Source: CAD feature listing. Evaluate the final solid. Frame: model axes, mm. A direction names the side the tool comes from. Round coordinates to 2 decimals unless told otherwise and drop trailing zeros. Answer in a Markdown table with one row per item. Add a question column.
```python
from build123d import *

# Parameters (mm, degrees)
ESQUISSE2_R                  = 39.5
BOSS_EXTRU_1_DEPTH           = 1
ESQUISSE4_R                  = 41.25
BOSS_EXTRU_2_DEPTH           = 1
ESQUISSE5_R                  = 42
BOSS_EXTRU_3_DEPTH           = 7
ESQUISSE6_R                  = 35
BOSS_EXTRU_4_DEPTH           = 7
BOSS_EXTRU_7_DEPTH           = 3
R_P_TITION_START             = -52
R_P_TITION_CIRCULAIRE1_DEPTH = 3
ESQUISSE8_R                  = 15
BOSS_EXTRU_8_DEPTH           = 10
ESQUISSE9_W                  = 24
ESQUISSE9_H                  = 40
BOSS_EXTRU_9_DEPTH           = 42
BOSS_EXTRU_10_DEPTH          = 24
ESQUISSE11_R                 = 15
BOSS_EXTRU_11_DEPTH          = 10
BOSS_EXTRU_12_START          = 10
ESQUISSE12_R                 = 15
BOSS_EXTRU_12_DEPTH          = 10


# Read off the part's stored shape, not the designer's step: Répétition circulaire1
with BuildPart() as part:
    # Esquisse1 → Révolution1 (revolve)
    with BuildSketch(Plane.XY):
        with BuildLine():
            Line((0, 0), (-35, 0))
            ThreePointArc((-35, 0), (-39.657515479, -9.46062113), (-40, -20))
            Line((-40, -20), (0, -20))
            Line((0, -20), (0, 0))
        make_face()
    revolve(axis=Axis((0, 0, 0), (0, -1, 0)))

    # Esquisse2 → Boss.-Extru.1 (add)
    with BuildSketch(Plane.XZ.offset(20)):
        Circle(ESQUISSE2_R)
    extrude(amount=BOSS_EXTRU_1_DEPTH)

    # Esquisse3 → Révolution2 (revolve)
    with BuildSketch(Plane(origin=(0, 0, 0), x_dir=(0, 0, -1), z_dir=(1, 0, 0)), mode=Mode.PRIVATE) as r_volution2_sk:
        with BuildLine():
            Line((0, -21), (-40, -21))
            ThreePointArc((-40, -21), (-42.384109041, -30.861589096), (-42, -41))
            Line((-42, -41), (0, -41))
            Line((0, -41), (0, -21))
        make_face()
    revolve(r_volution2_sk.sketch.rotate(Axis((0, -21, 0), (0, -1, 0)), 90), axis=Axis((0, -21, 0), (0, -1, 0)))

    # Esquisse4 → Boss.-Extru.2 (add)
    with BuildSketch(Plane.XZ.offset(41)):
        with Locations(Location((0, 0, 0), (0, 0, 270))):
            Circle(ESQUISSE4_R)
    extrude(amount=BOSS_EXTRU_2_DEPTH)

    # Esquisse5 → Boss.-Extru.3 (add)
    with BuildSketch(Plane.XZ.offset(42)):
        with Locations(Location((0, 0, 0), (0, 0, 270))):
            Circle(ESQUISSE5_R)
    extrude(amount=BOSS_EXTRU_3_DEPTH)

    # Esquisse6 → Boss.-Extru.4 (add)
    with BuildSketch(Plane.XZ.offset(49)):
        with Locations(Location((0, 0, 0), (0, 0, 270))):
            Circle(ESQUISSE6_R)
    extrude(amount=BOSS_EXTRU_4_DEPTH)

    # Esquisse7 → Boss.-Extru.7 (add)
    with BuildSketch(Plane.XZ.offset(49)):
        Polygon((39.629367086, -1.94603582), (40.75, 0.005042677), (39.620632914, 1.951078497), (37.370632914, 1.94603582), (36.25, -0.005042677), (37.379367086, -1.951078497), align=None)
        Polygon((39.045525279, 0.94978706), (37.950222917, 0.94733228), (37.404697638, -0.00245478), (37.954474721, -0.94978706), (39.049777083, -0.94733228), (39.595302362, 0.00245478), align=None, mode=Mode.SUBTRACT)
    extrude(amount=BOSS_EXTRU_7_DEPTH)

    # Répétition circulaire1 outline → Répétition circulaire1 (add)
    # profile 1 of 7: a face of its own
    with BuildSketch(Plane(origin=(0, 0, 0), x_dir=(1, 0, 0), z_dir=(0, 1, 0)).offset(R_P_TITION_START)):
        Polygon((29.398249326, -26.646139076), (27.810824779, -25.051583107), (25.636186529, -25.629055107), (25.048972826, -27.801083076), (26.636397373, -29.395639044), (28.811035623, -28.818167044), align=None)
        Polygon((28.282227258, -26.9424971), (27.996371011, -27.999842595), (26.937754829, -28.28095657), (26.164994893, -27.504725051), (26.45085114, -26.447379557), (27.509467323, -26.166265581), align=None, mode=Mode.SUBTRACT)
    # profile 2 of 7: a face of its own
    with BuildSketch(Plane(origin=(0, 0, 0), x_dir=(1, 0, 0), z_dir=(0, 1, 0)).offset(R_P_TITION_START)):
        Polygon((26.646139076, 29.398249326), (25.051583107, 27.810824779), (25.629055107, 25.636186529), (27.801083076, 25.048972826), (29.395639044, 26.636397373), (28.818167044, 28.811035623), align=None)
        Polygon((26.9424971, 28.282227258), (27.999842595, 27.996371011), (28.28095657, 26.937754829), (27.504725051, 26.164994893), (26.447379557, 26.45085114), (26.166265581, 27.509467323), align=None, mode=Mode.SUBTRACT)
    # profile 3 of 7: a face of its own
    with BuildSketch(Plane(origin=(0, 0, 0), x_dir=(1, 0, 0), z_dir=(0, 1, 0)).offset(R_P_TITION_START)):
        Polygon((-1.94603582, 39.629367086), (-1.951078497, 37.379367086), (-0.005042677, 36.25), (1.94603582, 37.370632914), (1.951078497, 39.620632914), (0.005042677, 40.75), align=None)
        Polygon((-0.94733228, 39.049777083), (0.00245478, 39.595302362), (0.94978706, 39.045525279), (0.94733228, 37.950222917), (-0.00245478, 37.404697638), (-0.94978706, 37.954474721), align=None, mode=Mode.SUBTRACT)
    # profile 4 of 7: a face of its own
    with BuildSketch(Plane(origin=(0, 0, 0), x_dir=(1, 0, 0), z_dir=(0, 1, 0)).offset(R_P_TITION_START)):
        Polygon((-29.398249326, 26.646139076), (-27.810824779, 25.051583107), (-25.636186529, 25.629055107), (-25.048972826, 27.801083076), (-26.636397373, 29.395639044), (-28.811035623, 28.818167044), align=None)
        Polygon((-28.282227258, 26.9424971), (-27.996371011, 27.999842595), (-26.937754829, 28.28095657), (-26.164994893, 27.504725051), (-26.45085114, 26.447379557), (-27.509467323, 26.166265581), align=None, mode=Mode.SUBTRACT)
    # profile 5 of 7: a face of its own
    with BuildSketch(Plane(origin=(0, 0, 0), x_dir=(1, 0, 0), z_dir=(0, 1, 0)).offset(R_P_TITION_START)):
        Polygon((-39.629367086, -1.94603582), (-37.379367086, -1.951078497), (-36.25, -0.005042677), (-37.370632914, 1.94603582), (-39.620632914, 1.951078497), (-40.75, 0.005042677), align=None)
        Polygon((-39.049777083, -0.94733228), (-39.595302362, 0.00245478), (-39.045525279, 0.94978706), (-37.950222917, 0.94733228), (-37.404697638, -0.00245478), (-37.954474721, -0.94978706), align=None, mode=Mode.SUBTRACT)
    # profile 6 of 7: a face of its own
    with BuildSketch(Plane(origin=(0, 0, 0), x_dir=(1, 0, 0), z_dir=(0, 1, 0)).offset(R_P_TITION_START)):
        Polygon((-26.646139076, -29.398249326), (-25.051583107, -27.810824779), (-25.629055107, -25.636186529), (-27.801083076, -25.048972826), (-29.395639044, -26.636397373), (-28.818167044, -28.811035623), align=None)
        Polygon((-26.9424971, -28.282227258), (-27.999842595, -27.996371011), (-28.28095657, -26.937754829), (-27.504725051, -26.164994893), (-26.447379557, -26.45085114), (-26.166265581, -27.509467323), align=None, mode=Mode.SUBTRACT)
    # profile 7 of 7: a face of its own
    with BuildSketch(Plane(origin=(0, 0, 0), x_dir=(1, 0, 0), z_dir=(0, 1, 0)).offset(R_P_TITION_START)):
        Polygon((1.94603582, -39.629367086), (1.951078497, -37.379367086), (0.005042677, -36.25), (-1.94603582, -37.370632914), (-1.951078497, -39.620632914), (-0.005042677, -40.75), align=None)
        Polygon((0.94733228, -39.049777083), (-0.00245478, -39.595302362), (-0.94978706, -39.045525279), (-0.94733228, -37.950222917), (0.00245478, -37.404697638), (0.94978706, -37.954474721), align=None, mode=Mode.SUBTRACT)
    extrude(amount=R_P_TITION_CIRCULAIRE1_DEPTH)

    # Esquisse8 → Boss.-Extru.8 (add)
    with BuildSketch(Plane.XZ.offset(56)):
        with Locations(Location((0, 0, 0), (0, 0, 270))):
            Circle(ESQUISSE8_R)
    extrude(amount=BOSS_EXTRU_8_DEPTH)

    # Esquisse9 → Boss.-Extru.9 (add)
    with BuildSketch(Plane(origin=(0, 0, 0), x_dir=(1, 0, 0), z_dir=(0, 1, 0))):
        Rectangle(ESQUISSE9_W, ESQUISSE9_H)
    extrude(amount=BOSS_EXTRU_9_DEPTH)

    # Esquisse10 → Boss.-Extru.10 (add)
    with BuildSketch(Plane.ZY.offset(12)):
        with BuildLine():
            Line((-20, 42), (20, 42))
            ThreePointArc((20, 42), (0, 62), (-20, 42))
        make_face()
    extrude(amount=-BOSS_EXTRU_10_DEPTH)

    # Esquisse11 → Boss.-Extru.11 (add)
    with BuildSketch(Plane(origin=(12, 0, 0), x_dir=(0, 0, -1), z_dir=(1, 0, 0))):
        with Locations(Location((0, 42, 0), (0, 0, 180))):
            Circle(ESQUISSE11_R)
    extrude(amount=BOSS_EXTRU_11_DEPTH)

    # Esquisse12 → Boss.-Extru.12 (add)
    with BuildSketch(Plane.ZY.offset(12).offset(BOSS_EXTRU_12_START)):
        with Locations((0, 42)):
            Circle(ESQUISSE12_R)
    extrude(amount=-BOSS_EXTRU_12_DEPTH)


solid = part.part
```
(1) Access query for faces 4 (the face through (26, -52, -27)), 5 (the face through (-40.27, -41.49, 8.94)), 6 (the face through (16.93, 27.128, -1.953)), 7 (the face through (39.5, -52, 0.5)), 8 (the face through (27, -52, 26)). Directions: +Z, -Z, +X, -X, +Y, -Y. A direction counts if a zero-diameter tool reaches every point of the face in a straight line with its end or side. Return the directions, or none.
(2) Draft query along Y for faces 1 (the face through (-17.07, 56.872, -1.953)), 2 (the face through (0, -66, 0)), 3 (the face through (22, 42, 0)). Return one class per face: +Y half, -Y half, draft (parallel to the pull), parting line (faces both ways), or undercut.
(3) Pin query (flat end, axial travel): pin 1 (10 mm diameter, centred on x = 24.5, y = 27.5, fed in from +Z); pin 2 (8 mm diameter, centred on y = 23, z = 4.5, fed in from +X); pin 3 (10 mm diameter, centred on y = 25.5, z = 3.5, fed in from +X). Return the tip coordinate at first contact, or that it passes through.
(4) Line query: line 1 (X direction, y = 6, z = -10.5); line 2 (Y direction, x = -18.5, z = 21.5); line 3 (Y direction, x = 18, z = -10.5). Output: solid intervals per line, ascending. Write a range as from..to.
Answer list:
| question | item | result |
|---|---|---|
| 1 | face 4 | -Z, +X, -Y |
| 1 | face 5 | none |
| 1 | face 6 | +X |
| 1 | face 7 | +Z, -Z, +X, -Y |
| 1 | face 8 | +Z, +X, -Y |
| 2 | face 1 | undercut |
| 2 | face 2 | -Y half |
| 2 | face 3 | draft |
| 3 | pin 1 | z = 11.03 |
| 3 | pin 2 | x = 12 |
| 3 | pin 3 | x = 22 |
| 4 | line 1 | -12..12 |
| 4 | line 2 | -56..0 |
| 4 | line 3 | -56..0, 31.29..52.71 |
